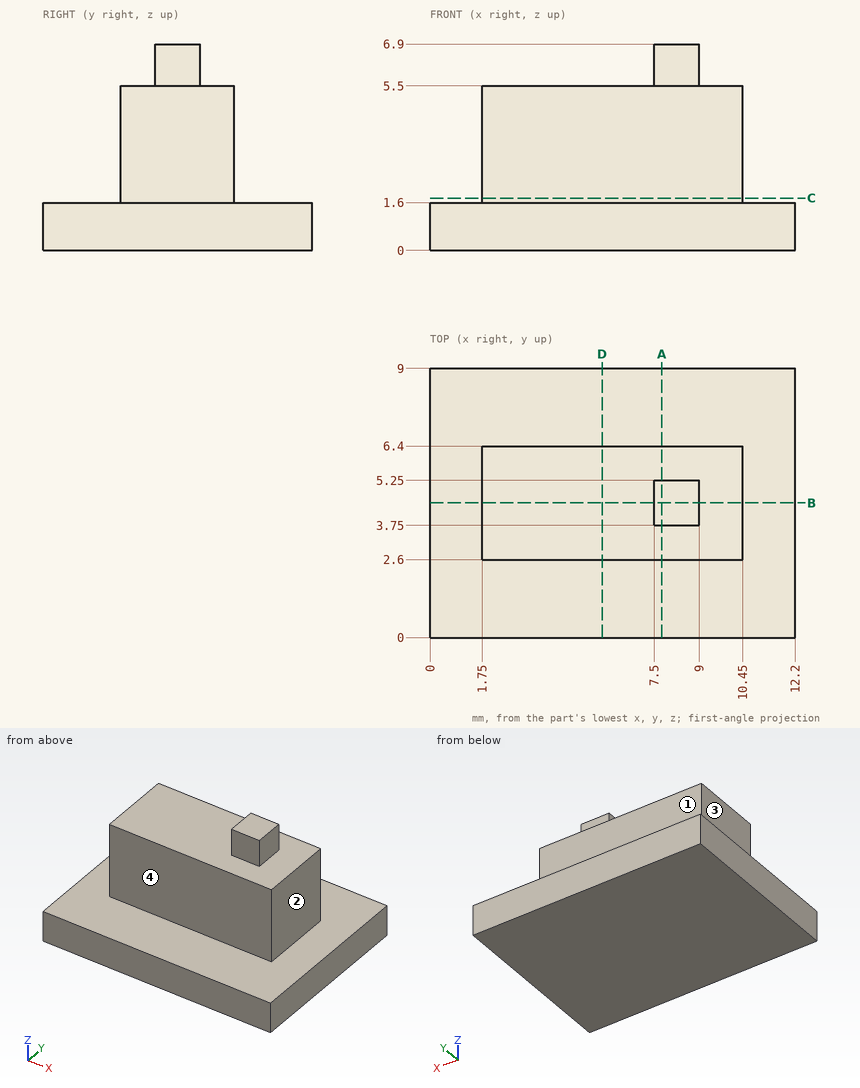
Study the drawing (mm; zero at the part's minimum x, y, z) and answer. A direction names the side the tool comes from. Give positions to 0.01 mm unless a question says otherwise; leave off trailing zeros. Loops run counter-clockwise (first coordinate to the right, second up) from the corner with the lowest first, then second, coordinate; pieces in that order, holes last. Notation, with made-up numbers: (77.25, 76.5) - (98.25, 76.5) arc R27 ccw to (98.25, 114.5) - close; hole circle Ø9 at (72.25, 44.5). An arc over 180 degrees is marked (long way). Return JSON: item names as keys, results as strings. Group by question number.
1. Find section A-A (x = 7.75). Write down the section's boundary in (y, z), then the cut area to 3 significant figures.
2. Which of the six approach directions +Z, -Z, +X, -X, +Y, -Y give full straight-line access (tool end or side, diameter ignored) to the marked faces 1, 2, 3 and 4?
3. Find section C-C (z = 1.75). Write down the section's boundary in (x, y).
4. Find section B-B (y = 4.5). Write down the section's boundary in (x, z), then the cut area to 4 significant figures.
5. Find section D-D (x = 5.75). Write down the section's boundary in (y, z), then the cut area to 3 significant figures.
6. Straight lines are drawn through the part: line 1 (Z direction, x = 5.25, y = 6.5); line 2 (Y direction, x = 6.75, z = 2); line 3 (Z direction, x = 8.5, y = 2.75). For each, find the intervals that lie inside material, in ascending order. Write a range as [from, to].
7. Given pin 1 Ø1.5 at (x, z) = (8.5, 6.5) entering from -Y; pin 2 Ø3 at (y, z) = (4.5, 4) entering from +X; pin 3 Ø1.5 at (x, z) = (8, 6.5) entering from +Y, each flat-ended and moving along its own axis, determine where each tip first touches the part or whether it passes through.
Verdict:
{
 "1": {"outline": "(0, 0) - (9, 0) - (9, 1.6) - (6.4, 1.6) - (6.4, 5.5) - (5.25, 5.5) - (5.25, 6.9) - (3.75, 6.9) - (3.75, 5.5) - (2.6, 5.5) - (2.6, 1.6) - (0, 1.6) - close", "area": "31.3 mm^2"},
 "2": {"face 1": "+Z, +X, -X, +Y", "face 2": "+Z, +X, +Y, -Y", "face 3": "+Z, -X, +Y, -Y", "face 4": "+Z, +X, -X, -Y"},
 "3": {"outline": "(1.75, 2.6) - (10.45, 2.6) - (10.45, 6.4) - (1.75, 6.4) - close"},
 "4": {"outline": "(0, 0) - (12.2, 0) - (12.2, 1.6) - (10.45, 1.6) - (10.45, 5.5) - (9, 5.5) - (9, 6.9) - (7.5, 6.9) - (7.5, 5.5) - (1.75, 5.5) - (1.75, 1.6) - (0, 1.6) - close", "area": "55.55 mm^2"},
 "5": {"outline": "(0, 0) - (9, 0) - (9, 1.6) - (6.4, 1.6) - (6.4, 5.5) - (2.6, 5.5) - (2.6, 1.6) - (0, 1.6) - close", "area": "29.2 mm^2"},
 "6": {"line 1": "z = [0, 1.6]", "line 2": "y = [2.6, 6.4]", "line 3": "z = [0, 5.5]"},
 "7": {"pin 1": "stops at y = 3.75", "pin 2": "stops at x = 10.45", "pin 3": "stops at y = 5.25"}
}
